Could you check a few things on this model? Use its own coordinates, in mm. Face numbers are marked on the shaded views. A direction names the side the tool comes from. Coordinates: 2 decimals unless noted, no trailing zeros. Loops run counter-clockwise (first coordinate to the right, second up) from the corner with the lowest first, then second, coordinate; pieces in that order, holes last. Notation, with made-up numbers: (43.25, 11.5) - (93.25, 11.5) arc R18 cw to (93.25, 30.5) - close; hole circle Ø11 at (67.25, -20). An arc over 180 degrees is marked (long way). One line per item, written item: value. Start each with the question number.
(1) I'm going to push flat-ended pins straight in: P1, Ø25, axis at x = -15, y = -26.5, coming from the +Z side; P2, Ø12, axis at y = 0.5, z = 16.5, coming from the +X side; P3, Ø1, axis at y = -18, z = 8.5, coming from the +X side. Where does each tip first touch, or does it pass through?
(2) If we section it at B-B on z = 68: Write out the boundary of the cut face in (x, y).
(3) On a 3-axis mill with a long thin cutter (end or side, diameter ignored), from which of +Z, -Z, +X, -X, +Y, -Y can I reach the whole of each face in a straight line? I mean the marked faces 4, 5 and 6. Say none if no direction works.
(4) If I drill on line 1 along Z through (x, y) = (-5, 18); line 2 along X through (y, z) = (4.5, 65.5); line 3 along Y through (x, z) = (-20, 40), over which ranges is the centre line in solid material (lowest first)? Write a range as from..to.
(5) If we section it at C-C on z = 45: Write out the boundary of the cut face in (x, y), then the cut area to 3 significant figures.
(6) If we mould it in two halves opening along Y, with no side actions, what happens to the marked faces 1, 2 and 3? For each: pulls with the +Y half, pulls with the -Y half, needs draft (parallel to the pull), parting line crosses it, or undercut.
(7) If we section it at A-A on x = 0: Write out the boundary of the cut face in (y, z), then the cut area to 3 significant figures.
```python
from build123d import *

# Parameters (mm, degrees)
F0_W     = 75
F0_H     = 100
F1_DEPTH = 50


with BuildPart() as f1:
    # F0 (on Top) → F1 (new body)
    with BuildSketch(Plane.XY):
        Rectangle(F0_W, F0_H)
    extrude(amount=-F1_DEPTH)

    # F2 (on Right) → F3 (revolve)
    with BuildSketch(Plane.YZ):
        Polygon((-35.5, 0), (-20, 93.500273), (-22, 93.500273), (-37.5, 0), align=None)
    revolve(axis=Axis((0, 0, 46.750137), (0, 0, 1)))


solid = f1.part
```
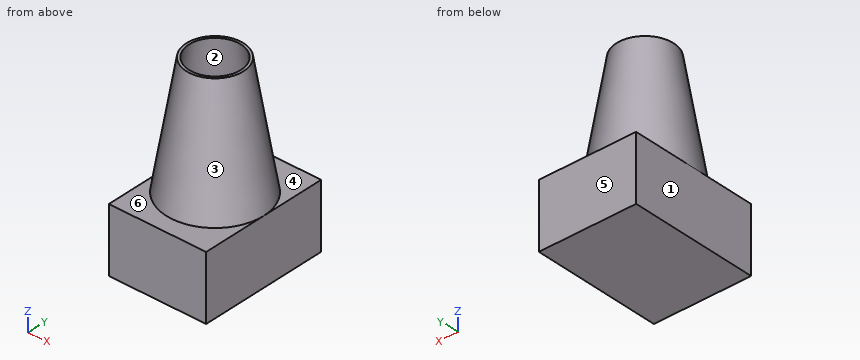
Values:
1. P1: stops at z = 93.5
1. P2: stops at x = 35.76
1. P3: stops at x = 31.58
2. outline: circle Ø52.45 at (0, 0); hole circle Ø48.45 at (0, 0)
3. face 4: +Z, +Y
3. face 5: +Z, -Z, +X, -X, +Y
3. face 6: +Z, -Y
4. line 1: z = -50..0
4. line 2: x = -26.26..-24.23, 24.23..26.26
4. line 3: y = -23.51..-20.82, 20.82..23.51
5. outline: circle Ø60.08 at (0, 0); hole circle Ø56.08 at (0, 0)
5. area: 365 mm2
6. face 1: needs draft
6. face 2: undercut
6. face 3: parting line crosses it
7. outline: (-50, -50) - (50, -50) - (50, 0) - (37.5, 0) - (22, 93.5) - (20, 93.5) - (35.5, 0) - (-35.5, 0) - (-20, 93.5) - (-22, 93.5) - (-37.5, 0) - (-50, 0) - close
7. area: 5,370 mm2
